The drawing under review shows one solid part. Ordinate dimensions are in mm from its lowest x, y, z. A direction names the side the tool comes from. Coordinates: 2 decimals unless noted, no trailing zeros. Write each loop counter-clockwise with the first axis right and the second up, starting at its lowest first coordinate (ties: lowest second). Pieces come first, ordered by that corner, then holes.
1) We need section B-B on y = 4. Write out the cut boundary in (x, z) (3 decimals), then the cut area to 3 significant figures.
2) We need section A-A on x = 8. Write out the cut boundary in (y, z) (3 decimals), then the cut area to 3 significant figures.
3) Mouldability with a two-part tool opening along Y and no side actions: class the marked faces 4, 5, 6 and 7 as pulls with the +Y half, pulls with the -Y half, needs draft (parallel to the pull), parting line crosses it, or undercut.
4) We need section D-D on y = 13.25. Write out the cut boundary in (x, z).
5) We need section C-C on x = 4. Write out the cut boundary in (y, z) (3 decimals), then the cut area to 3 significant figures.
6) For the marked faces 1, 2 and 3, list the 3-axis set-ups (+Z, -Z, +X, -X, +Y, -Y) from which the entire face can be reached by the end or side of a thin tool; tool diameter is ignored.
7) To check wall thickness, follow line 1 along Y through (x, z) = (20.5, 2.5); line 2 along Y through (x, z) = (25, 4); line 3 along Y through (x, z) = (24, 1) (3 decimals). State the ranges of each line that lie inside material, in increasing order.
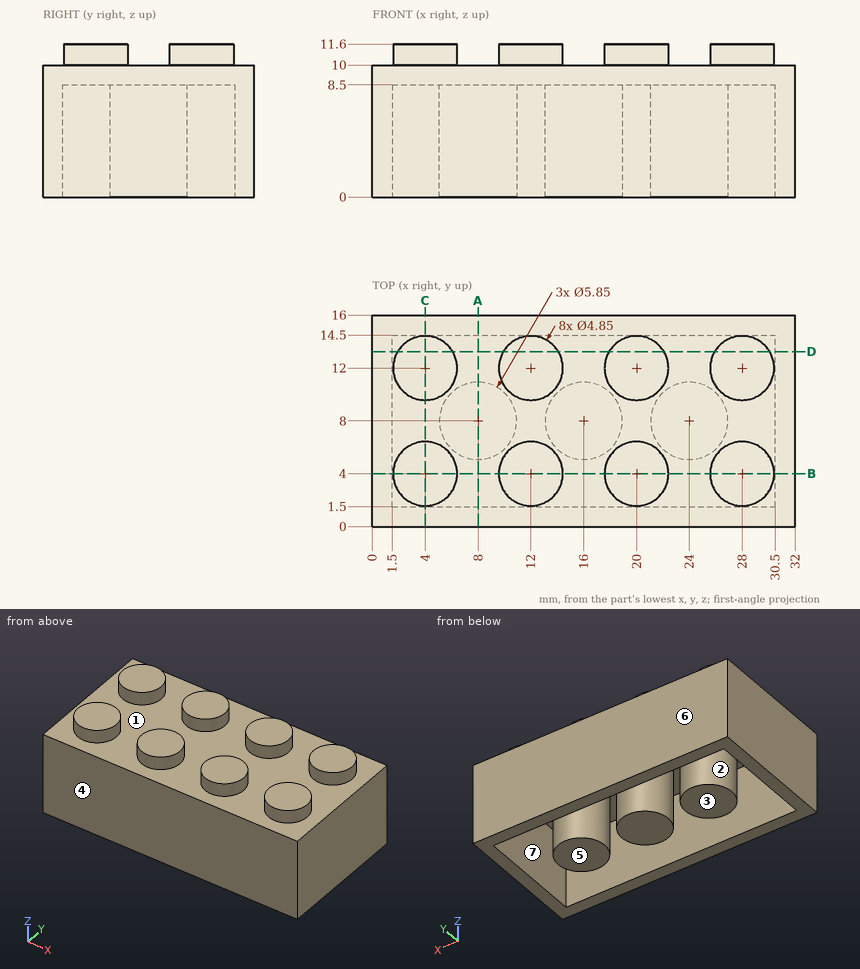
Result:
1. outline: (0, 0) - (1.5, 0) - (1.5, 8.5) - (30.5, 8.5) - (30.5, 0) - (32, 0) - (32, 10) - (30.425, 10) - (30.425, 11.6) - (25.575, 11.6) - (25.575, 10) - (22.425, 10) - (22.425, 11.6) - (17.575, 11.6) - (17.575, 10) - (14.425, 10) - (14.425, 11.6) - (9.575, 11.6) - (9.575, 10) - (6.425, 10) - (6.425, 11.6) - (1.575, 11.6) - (1.575, 10) - (0, 10) - close
1. area: 105 mm2
2. outline: (0, 0) - (1.5, 0) - (1.5, 8.5) - (5.075, 8.5) - (5.075, 0) - (10.925, 0) - (10.925, 8.5) - (14.5, 8.5) - (14.5, 0) - (16, 0) - (16, 10) - (0, 10) - close
2. area: 99.2 mm2
3. face 4: pulls with the -Y half
3. face 5: needs draft
3. face 6: pulls with the +Y half
3. face 7: undercut
4. outline: (0, 0) - (1.5, 0) - (1.5, 8.5) - (30.5, 8.5) - (30.5, 0) - (32, 0) - (32, 10) - (30.08, 10) - (30.08, 11.6) - (25.92, 11.6) - (25.92, 10) - (22.08, 10) - (22.08, 11.6) - (17.92, 11.6) - (17.92, 10) - (14.08, 10) - (14.08, 11.6) - (9.92, 11.6) - (9.92, 10) - (6.08, 10) - (6.08, 11.6) - (1.92, 11.6) - (1.92, 10) - (0, 10) - close
5. outline: (0, 0) - (1.5, 0) - (1.5, 8.5) - (14.5, 8.5) - (14.5, 0) - (16, 0) - (16, 10) - (14.425, 10) - (14.425, 11.6) - (9.575, 11.6) - (9.575, 10) - (6.425, 10) - (6.425, 11.6) - (1.575, 11.6) - (1.575, 10) - (0, 10) - close
5. area: 65.0 mm2
6. face 1: +Z
6. face 2: -Z
6. face 3: -Z, +X, -X, +Y, -Y
7. line 1: y = 0 to 1.5, 14.5 to 16
7. line 2: y = 0 to 1.5, 5.25 to 10.75, 14.5 to 16
7. line 3: y = 0 to 1.5, 5.075 to 10.925, 14.5 to 16
